Autodesk Inventor part; units mm, degrees
ref_plane "YZ Plane" through (0, 0, 0) normal (1, 0, 0) x (0, 1, 0)
ref_plane "XZ Plane" through (0, 0, 0) normal (0, 1, 0) x (-1, 0, 0)
ref_plane "XY Plane" through (0, 0, 0) normal (0, 0, 1) x (1, 0, 0)
sketch "Sketch1" plane through (0, 0, 0) normal (0, 0, 1) x (1, 0, 0)
  line L0 (14.9983, 97.5) -> (14.9983, -62.4997)
  line L1 (14.9983, -62.4997) -> (-15, -62.5003)
  line L2 (-15, -62.5003) -> (-15, 97.7282)
  circle A0 centre (-0.0017, 97.5) radius 3.2
  circle A1 centre (9.9983, -58.4998) radius 2
  circle A2 centre (-10, -58.5002) radius 2
  arc A3 (14.9983, 97.5) -> (-15, 97.7282) centre (-0.0017, 97.5) ccw
  point P0 (0, 0)
  point P1 (-4.1636, 111.9111)
  point P2 (4.161, 111.9108)
  dimension "d2" = 62.5
  dimension "d3" = 15
  dimension "d4" = 6.4
  dimension "d5" = 15
  dimension "d7" = 4
  dimension "d8" = 4
  dimension "d9" = 5
  dimension "d10" = 4
  dimension "d11" = 4
  dimension "d12" = 5
  dimension "d17" = 160
extrude "Extrusion1" add sketch "Sketch1" along normal blind 10
equation "\"d5\" = 0.5 * d1"
equation "\"d11\" = d10"
equation "\"d12\" = d9"
properties part number "spool arm support"
Source: CAD feature listing. Evaluate the final solid. Frame: model axes, mm. Round coordinates to 2 decimals unless told otherwise and drop trailing zeros. Write each loop counter-clockwise with the first axis right and the second up, starting at its lowest first coordinate (ties: lowest second). Pieces come first, ordered by that corner, then holes. Notation, with made-up numbers: (45, 70) - (49, 70) arc R23 ccw to (49, 90) - close; hole circle Ø3 at (83, 88). An arc over 180 degrees is marked (long way). Use CSV: the item, a comma, the result in double quotes. Start each with the question number.
(1) Material intervals for probe 1 along Y at (x, z) = (-8.25, 8.75); probe 2 along Y at (x, z) = (-2.5, 3); probe 3 along Y at (x, z) = (-7.25, 7.25), sorted ascending. Write a range as [from, to].
(2) Cut plane B-B, the plane z = 3. Return loops of the section in (x, y).
(3) First-contact query: pin 1 Ø5 at (x, z) = (-2, 8) entering from +Y; pin 2 Ø1.5 at (x, z) = (-6, 3.5) entering from +Y; pin 3 Ø3 at (x, z) = (-11, 8) entering from +Y. Flat tips, straight axial feed; report the tip coordinate or a pass-through.
(4) Mould query, pull axis X, two halves, no side actions, for faces 1 (the face through (0, 26, 0)), 2 (the face through (10.921, -56.725, 4.93)), 3 (the face through (-0.2, 112.5, 4.9)). Classes: pulls with the +X half, pulls with the -X half, needs draft (parallel to the pull), parting line crosses it, or undercut.
(5) Cut plane A-A, the plane x = -10. Return loops of the section in (y, z), and give its area (3 significant figures).
Geometry says:
1,probe 1,"[-62.5, -59.47], [-57.53, 110.03]"
1,probe 2,"[-62.5, 95.5], [99.5, 112.29]"
1,probe 3,"[-62.5, 110.63]"
2,outline,"(-15, -62.5) - (15, -62.5) - (15, 97.5) arc R15 ccw to (-15, 97.73) - close; hole circle Ø4 at (-10, -58.5); hole circle Ø6.4 at (0, 97.5); hole circle Ø4 at (10, -58.5)"
3,pin 1,"y = 112.5"
3,pin 2,"y = 111.55"
3,pin 3,"y = 109.11"
4,face 1,"needs draft"
4,face 2,"undercut"
4,face 3,"parting line crosses it"
5,outline,"(-62.5, 0) - (-60.5, 0) - (-60.5, 10) - (-62.5, 10) - close; (-56.5, 0) - (108.68, 0) - (108.68, 10) - (-56.5, 10) - close"
5,area,"1,670 mm²"
